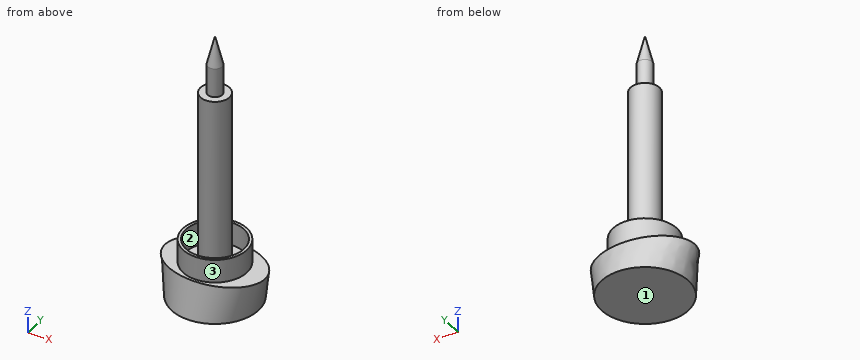
Autodesk Inventor part; units mm, degrees
ref_plane "Work Plane1" through (0, 0, 6) normal (0, 0, 1) x (1, 0, 0)
ref_plane "Work Plane2" through (0, 0, 46) normal (0, 0, 1) x (1, 0, 0)
ref_plane "YZ Plane" through (0, 0, 0) normal (1, 0, 0) x (0, 1, 0)
sketch "Sketch1" plane through (0, 0, 0) normal (0, 0, 1) x (1, 0, 0)
  circle A0 centre (0, 0) radius 7.5
  dimension "d0" = 15
ref_plane "Work Plane1" through (0, 0, 6) normal (0, 0, 1) x (1, 0, 0)
sketch "Sketch2" plane through (0, 0, 6) normal (0, 0, 1) x (1, 0, 0)
  ellipse E0 centre (0, 0) end of major axis (8.6502, 0) minor radius 6
  line L0 (0, 0) -> (-7.5, 0)
  dimension "d26" = 7.5
loft "Loft1" add profiles "Sketch1", "Sketch2"
sketch "Sketch3" plane through (0, 0, 6) normal (0, 0, 1) x (1, 0, 0)
  circle A0 centre (0, 0) radius 5
  circle A1 centre (0, 0) radius 5.5
  dimension "d11" = 10
  dimension "d12" = 11
extrude "Extrusion2" add sketch "Sketch3" along normal blind 4
sketch "Sketch4" plane through (0, 0, 6) normal (0, 0, 1) x (1, 0, 0)
  circle A0 centre (0, 0) radius 2.5
  dimension "d15" = 5
extrude "Extrusion3" add sketch "Sketch4" along normal blind 30
sketch "Sketch5" plane through (0, 0, 36) normal (0, 0, 1) x (1, 0, 0)
  circle A0 centre (0, 0) radius 1.25
  dimension "d18" = 2.5
extrude "Extrusion4" add sketch "Sketch5" along normal blind 5
sketch "Sketch6" plane through (0, 0, 41) normal (0, 0, 1) x (1, 0, 0)
  point P0 (0, 0)
ref_plane "Work Plane2" through (0, 0, 46) normal (0, 0, 1) x (1, 0, 0)
sketch "Sketch7" plane through (0, 0, 46) normal (0, 0, 1) x (1, 0, 0)
  point P0 (0, 0)
  point P1 (0, 0)
loft "Loft2" add section 1 edges at (-1.25, 0, 41) section 2 point at (0, 0, 46)
properties part number "Solder"
Here's how the part is built. I have some questions about the finished solid (model axes, mm). Face numbers are marked on the shaded views. Coordinates: 2 decimals unless noted, no trailing zeros. Loops run counter-clockwise (first coordinate to the right, second up) from the corner with the lowest first, then second, coordinate; pieces in that order, holes last. Notation, with made-up numbers: (58, -33) - (102, -33) arc R16 ccw to (102, -11) - close; hole circle Ø10 at (62.5, 10.5). An arc over 180 degrees is marked (long way). Return JSON: item names as keys, results as strings. Group by question number.
Item 1: If we section it at B-B on z = 14.5: Write out the boundary of the cut face in (x, y).
Item 2: If we section it at A-A on z = 40: Write out the boundary of the cut face in (x, y).
Item 3: I need wall thicknesses on line 1 (Y direction, x = 0, z = 8.3); line 2 (Z direction, x = -1.5, y = -5.75); line 3 (Z direction, x = 1.25, y = 5). Which ranges of each line are inside material? Lowest first, please. Write a range as from..to.
Item 4: Will these pins go through, and if not, where does the flat tip stop? P1, Ø3, axis at x = 1.5, z = 19.5, coming from the -Y side; P2, Ø8, axis at y = 3.5, z = 7, coming from the -X side; P3, Ø4, axis at y = 1.5, z = 34, coming from the -X side; P4, Ø6, axis at y = 5, z = 5.5, coming from the -X side.
Item 5: We'd pull the mould along X, two halves only. Please class the marked faces 1, 2 and 3: +X half, -X half, draft (parallel to the pull), parting line (faces both ways), or undercut.
Calculated:
{
 "1": {"outline": "circle Ø5 at (0, 0)"},
 "2": {"outline": "circle Ø2.5 at (0, 0)"},
 "3": {"line 1": "y = -5.5..-5, -2.5..2.5, 5..5.5", "line 2": "z = 0..6", "line 3": "z = 0..10"},
 "4": {"P1": "stops at y = -2.5", "P2": "stops at x = -8.65", "P3": "stops at x = -2.5", "P4": "stops at x = -8.13"},
 "5": {"face 1": "draft", "face 2": "undercut", "face 3": "parting line"}
}
